from build123d import *

# Parameters (mm, degrees)
SKETCH1_R               = 12.5
BOSS_EXTRUDE1_DEPTH     = 40
SKETCH2_R               = 11.5
BOSS_EXTRUDE2_DEPTH     = 2
SKETCH3_R               = 11.5
BOSS_EXTRUDE3_DEPTH     = 2
SKETCH4_R               = 2.5
CUT_EXTRUDE1_DEPTH      = 1
CUT_EXTRUDE1_DEPTH_BACK = 45


with BuildPart() as part:
    # Sketch1 → Boss-Extrude1 (new body)
    with BuildSketch(Plane(origin=(0, 0, 0), x_dir=(1, 0, 0), z_dir=(0, 1, 0))):
        Circle(SKETCH1_R)
    extrude(amount=BOSS_EXTRUDE1_DEPTH)

    # Sketch2 → Boss-Extrude2 (add)
    with BuildSketch(Plane(origin=(0, 40, 0), x_dir=(1, 0, 0), z_dir=(0, 1, 0))):
        Circle(SKETCH2_R)
    extrude(amount=BOSS_EXTRUDE2_DEPTH)

    # Sketch3 → Boss-Extrude3 (add)
    with BuildSketch(Plane.XZ):
        Circle(SKETCH3_R)
    extrude(amount=BOSS_EXTRUDE3_DEPTH)

    # Sketch4 → Cut-Extrude1 (cut, two sides)
    with BuildSketch(Plane(origin=(0, -2, 0), x_dir=(-1, 0, 0), z_dir=(0, -1, 0))) as cut_extrude1_sk:
        Circle(SKETCH4_R)
    extrude(amount=CUT_EXTRUDE1_DEPTH, mode=Mode.SUBTRACT)
    extrude(cut_extrude1_sk.sketch, amount=-CUT_EXTRUDE1_DEPTH_BACK, mode=Mode.SUBTRACT)


solid = part.part
Work out the finished part from the listing and answer in its coordinate system (mm). A direction names the side the tool comes from. Give positions to 0.01 mm unless a question says otherwise; leave off trailing zeros. Write each loop counter-clockwise with the first axis right and the second up, starting at its lowest first coordinate (ties: lowest second). Pieces come first, ordered by that corner, then holes.
Q1. The part is cut by section D-D on y = 24. Give the vertices of the cut face in (x, z).
Answer:
outline: circle Ø25 at (0, 0); hole circle Ø5 at (0, 0)
Q2. For a pull along Z with two mould halves and no side action, classify faces 4 (the face through (0, 42, -3)), 5 (the face through (-1.5, -1, 11.4)), 6 (the face through (0.54, 19.69, 2.44)) as released by +Z, released by -Z, zero draft, split by the parting line, or undercut.
Answer:
face 4: zero draft
face 5: split by the parting line
face 6: undercut
Q3. Given pin 1 (4.5 mm diameter, centred on x = 0, z = 0, fed in from +Y); pin 2 (4 mm diameter, centred on y = 29, z = -4, fed in from -X); pin 3 (1 mm diameter, centred on x = -5, y = 27, fed in from -Z); pin 4 (4 mm diameter, centred on y = 32, z = 7.5, fed in from +X) (3 decimals), each flat-ended and moving along its own axis, determine where each tip first touches the part or whether it passes through.
Answer:
pin 1: passes through
pin 2: stops at x = -12.34
pin 3: stops at z = -11.66
pin 4: stops at x = 11.225
Q4. The part is cut by section A-A on z = 0. Give the vertices of the cut face in (x, y), and give its area (3 significant figures).
Answer:
outline: (-12.5, 0) - (-11.5, 0) - (-11.5, -2) - (-2.5, -2) - (-2.5, 42) - (-11.5, 42) - (-11.5, 40) - (-12.5, 40) - close; (2.5, -2) - (11.5, -2) - (11.5, 0) - (12.5, 0) - (12.5, 40) - (11.5, 40) - (11.5, 42) - (2.5, 42) - close
area: 872 mm2
Q5. Straight lines are drawn through the part: L1, parallel to Z at x = 0, y = 16; L2, parallel to Z at x = -1, y = 11. For each, find the intervals that lie inside material, in ascending order.
Answer:
L1: z = -12.5 to -2.5, 2.5 to 12.5
L2: z = -12.46 to -2.29, 2.29 to 12.46
Q6. The part is cut by section C-C on x = -4.75. Give the vertices of the cut face in (y, z), and give its area (3 significant figures).
Answer:
outline: (-2, -10.47) - (0, -10.47) - (0, -11.56) - (40, -11.56) - (40, -10.47) - (42, -10.47) - (42, 10.47) - (40, 10.47) - (40, 11.56) - (0, 11.56) - (0, 10.47) - (-2, 10.47) - close
area: 1,010 mm2
Q7. A tool of negligible diameter and unlimited length cuts with its end or side. For faces 1 (the face through (-1.5, 41, -11.4)), 2 (the face through (0, -2, 3)), 3 (the face through (11, 0, 4)), from which of +Z, -Z, +X, -X, +Y, -Y can it reach the whole face along a straight path? Write none if from no direction.
Answer:
face 1: +Y
face 2: +Z, -Z, +X, -X, -Y
face 3: -Y
Q8. The part is cut by section B-B on x = 0. Give the vertices of the cut face in (y, z).
Answer:
outline: (-2, -11.5) - (0, -11.5) - (0, -12.5) - (40, -12.5) - (40, -11.5) - (42, -11.5) - (42, -2.5) - (-2, -2.5) - close; (-2, 2.5) - (42, 2.5) - (42, 11.5) - (40, 11.5) - (40, 12.5) - (0, 12.5) - (0, 11.5) - (-2, 11.5) - close
